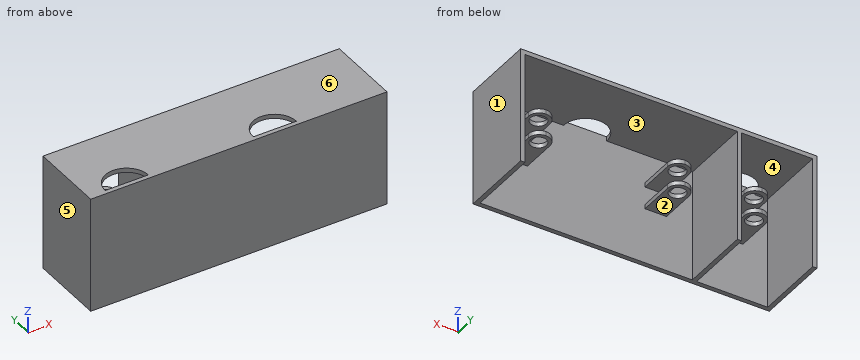
from build123d import *

# Parameters (mm, degrees)
BOSS_EXTRU_1_DEPTH      = 53.6
BOSS_EXTRU_1_DEPTH_BACK = 0.0001
ESQUISSE1_W             = 102.6
ESQUISSE1_H             = 35
ESQUISSE4_W             = 98.6
ESQUISSE4_H             = 51.6
ENL_V_MAT_EXTRU_2_DEPTH = 33
ESQUISSE9_W             = 10
ESQUISSE9_H             = 2
BOSS_EXTRU_3_DEPTH      = 21.5
CONG_2_R                = 5
ESQUISSE10_R            = 3.75
ENL_V_MAT_EXTRU_4_DEPTH = 15
ESQUISSE16_W            = 53.6001
ESQUISSE16_H            = 35
BOSS_EXTRU_5_DEPTH      = 35
ENL_V_MAT_EXTRU_5_DEPTH = 2.1
ESQUISSE19_W            = 33
ESQUISSE19_H            = 51.6001
ENL_V_MAT_EXTRU_6_DEPTH = 33
ENL_V_MAT_EXTRU_7_DEPTH = 2.5
ESQUISSE21_W            = 10
ESQUISSE21_H            = 2
BOSS_EXTRU_6_DEPTH      = 21.75
CONG_3_R                = 5
ESQUISSE22_R            = 3.75
ENL_V_MAT_EXTRU_8_DEPTH = 15


with BuildPart() as part:
    # Esquisse1 → Boss.-Extru.1 (new, two sides: drawn at the far end of the back side and taken through both)
    with BuildSketch(Plane.XY.offset(-BOSS_EXTRU_1_DEPTH_BACK)):
        with Locations((33.832170394, 1.686746988)):
            Rectangle(ESQUISSE1_W, ESQUISSE1_H)
    extrude(amount=BOSS_EXTRU_1_DEPTH + BOSS_EXTRU_1_DEPTH_BACK)

    # Esquisse4 → Enlèv. mat.-Extru.2 (cut)
    with BuildSketch(Plane(origin=(0, 19.186746988, 0), x_dir=(1, 0, 0), z_dir=(0, 1, 0))):
        with Locations((33.832170394, -25.7999)):
            Rectangle(ESQUISSE4_W, ESQUISSE4_H)
    extrude(amount=-ENL_V_MAT_EXTRU_2_DEPTH, mode=Mode.SUBTRACT)

    # Esquisse9 → Boss.-Extru.3 (add)
    with BuildSketch(Plane(origin=(0, -13.813253012, 0), x_dir=(1, 0, 0), z_dir=(0, 1, 0))):
        with Locations((1.532170394, -26.8499)):
            Rectangle(ESQUISSE9_W, ESQUISSE9_H)
        with Locations((1.532170394, -37.2299)):
            Rectangle(ESQUISSE9_W, ESQUISSE9_H)
        with Locations((66.132170394, -26.8499)):
            Rectangle(ESQUISSE9_W, ESQUISSE9_H)
        with Locations((66.132170394, -37.2299)):
            Rectangle(ESQUISSE9_W, ESQUISSE9_H)
    extrude(amount=BOSS_EXTRU_3_DEPTH)

    # Congé2
    cong_2_edges = [part.edges().sort_by_distance(p)[0] for p in [
        (71.132170394, 7.686746988, 37.2299),
        (61.132170394, 7.686746988, 37.2299),
        (71.132170394, 7.686746988, 26.8499),
        (61.132170394, 7.686746988, 26.8499),
        (-3.467829606, 7.686746988, 37.2299),
        (6.532170394, 7.686746988, 37.2299),
        (-3.467829606, 7.686746988, 26.8499),
        (6.532170394, 7.686746988, 26.8499),
    ]]
    fillet(cong_2_edges, radius=CONG_2_R - 0.0001)  # a hair under: the kernel refuses the full size

    # Esquisse10 → Enlèv. mat.-Extru.4 (cut)
    with BuildSketch(Plane(origin=(0, 0, 25.8499), x_dir=(-1, 0, 0), z_dir=(0, 0, -1))):
        with Locations((-66.132170394, 2.186746988)):
            Circle(ESQUISSE10_R)
        with Locations((-1.532170394, 2.186746988)):
            Circle(ESQUISSE10_R)
    extrude(amount=-ENL_V_MAT_EXTRU_4_DEPTH, mode=Mode.SUBTRACT)

    # Esquisse16 → Boss.-Extru.5 (add)
    with BuildSketch(Plane.ZY.offset(17.467829606)):
        with Locations((26.79995, 1.686746988)):
            Rectangle(ESQUISSE16_W, ESQUISSE16_H)
    extrude(amount=BOSS_EXTRU_5_DEPTH)

    # Esquisse18 → Enlèv. mat.-Extru.5 (cut)
    with BuildSketch(Plane.XY.offset(53.6)):
        with BuildLine():
            Line((24.333519225, -13.813253012), (44.330821563, -13.813253012))
            ThreePointArc((44.330821563, -13.813253012), (34.332170394, -3.643205178), (24.333519225, -13.813253012))
        make_face()
    extrude(amount=-ENL_V_MAT_EXTRU_5_DEPTH, mode=Mode.SUBTRACT)

    # Esquisse19 → Enlèv. mat.-Extru.6 (cut)
    with BuildSketch(Plane(origin=(0, 19.186746988, 0), x_dir=(1, 0, 0), z_dir=(0, 1, 0))):
        with Locations((-33.967829606, -25.79995)):
            Rectangle(ESQUISSE19_W, ESQUISSE19_H)
    extrude(amount=-ENL_V_MAT_EXTRU_6_DEPTH, mode=Mode.SUBTRACT)

    # Esquisse20 → Enlèv. mat.-Extru.7 (cut)
    with BuildSketch(Plane.XY.offset(53.6)):
        with BuildLine():
            Line((-24.467829606, -13.813253012), (-44.467829606, -13.813253012))
            ThreePointArc((-44.467829606, -13.813253012), (-34.467829606, -3.813253012), (-24.467829606, -13.813253012))
        make_face()
    extrude(amount=-ENL_V_MAT_EXTRU_7_DEPTH, mode=Mode.SUBTRACT)

    # Esquisse21 → Boss.-Extru.6 (add)
    with BuildSketch(Plane(origin=(0, -13.813253012, 0), x_dir=(1, 0, 0), z_dir=(0, 1, 0))):
        with Locations((-33.967829606, -26.8499)):
            Rectangle(ESQUISSE21_W, ESQUISSE21_H)
        with Locations((-33.967829606, -37.2299)):
            Rectangle(ESQUISSE21_W, ESQUISSE21_H)
    extrude(amount=BOSS_EXTRU_6_DEPTH)

    # Congé3
    cong_3_edges = [part.edges().sort_by_distance(p)[0] for p in [
        (-28.967829606, 7.936746988, 37.2299),
        (-38.967829606, 7.936746988, 37.2299),
        (-38.967829606, 7.936746988, 26.8499),
        (-28.967829606, 7.936746988, 26.8499),
    ]]
    fillet(cong_3_edges, radius=CONG_3_R - 0.0001)  # a hair under: the kernel refuses the full size

    # Esquisse22 → Enlèv. mat.-Extru.8 (cut)
    with BuildSketch(Plane(origin=(0, 0, 25.8499), x_dir=(-1, 0, 0), z_dir=(0, 0, -1))):
        with Locations((33.967829606, 2.186746988)):
            Circle(ESQUISSE22_R)
    extrude(amount=-ENL_V_MAT_EXTRU_8_DEPTH, mode=Mode.SUBTRACT)


solid = part.part
Could you check a few things on this model? Use its own coordinates, in mm. Face numbers are marked on the shaded views. A direction names the side the tool comes from. Give positions to 0.01 mm unless a question says otherwise; leave off trailing zeros. Loops run counter-clockwise (first coordinate to the right, second up) from the corner with the lowest first, then second, coordinate; pieces in that order, holes last. Notation, with made-up numbers: M 89.5,38 L 99.5,38 A24 ccw 99.5,75 Z; hole C -31.75,3 d1. An arc over 180 degrees is marked long. Answer as a JSON object with one key per item and string values.
Q1. Suppose I cut it at B-B, the plane z = 49. List the corners of the cut face in (x, y) for me, plus the area to 3 significant figures.
Values found:
{"outline": "M -52.47,-15.81 L 85.13,-15.81 L 85.13,19.19 L 83.13,19.19 L 83.13,-13.81 L -15.47,-13.81 L -15.47,19.19 L -17.47,19.19 L -17.47,-13.81 L -50.47,-13.81 L -50.47,19.19 L -52.47,19.19 Z", "area": "473 mm²"}
Q2. For P1, Ø3, axis at x = 68.5, y = -7, coming from the -Z side; P2, Ø1, axis at x = 51, y = -9, coming from the -Z side; P3, Ø5, axis at x = 48, z = 9.5, coming from the +Y side, each with a flat end and sliding along its axis, tell me the tip position at first contact or that it passes through.
Values found:
{"P1": "stops at z = 25.85", "P2": "stops at z = 51.6", "P3": "stops at y = -13.81"}
Q3. If I drill on probe 1 along X at (y, z) = (12, 46.5); probe 2 along Z at (x, y) = (6, 1.5); probe 3 along Z at (x, y) = (55.5, -3), over which ranges is the centre line in solid material (lowest first)? Write a range as [from, to].
Values found:
{"probe 1": "x = [-52.47, -50.47], [-17.47, -15.47], [83.13, 85.13]", "probe 2": "z = [25.85, 27.85], [36.23, 38.23], [51.6, 53.6]", "probe 3": "z = [51.6, 53.6]"}
Q4. For the marked faces 1 and 2, which set-ups out of +Z, -Z, +X, -X, +Y, -Y let a thin tool reach every point of the face, with its end or its side?
Values found:
{"face 1": "+Z, -Z, +X, +Y, -Y", "face 2": "-Z, +Y"}
Q5. Suppose I cut it at D-D, the plane x = 3.5. List the corners of the cut face in (y, z) for me, plus the area to 3 significant figures.
Values found:
{"outline": "M -15.81,0 L -13.81,0 L -13.81,25.85 L -1.01,25.85 L -1.01,27.85 L -13.81,27.85 L -13.81,36.23 L -1.01,36.23 L -1.01,38.23 L -13.81,38.23 L -13.81,51.6 L 19.19,51.6 L 19.19,53.6 L -15.81,53.6 Z; M 5.38,25.85 L 7.28,25.85 L 7.28,27.85 L 5.38,27.85 Z; M 5.38,36.23 L 7.28,36.23 L 7.28,38.23 L 5.38,38.23 Z", "area": "232 mm²"}
Q6. If we mould it in two halves opening along X, with no side actions, what happens to the marked faces 3, 4, 5 and 6? For each: pulls with the +X half, pulls with the -X half, needs draft (parallel to the pull), parting line crosses it, or undercut.
Values found:
{"face 3": "undercut", "face 4": "undercut", "face 5": "pulls with the -X half", "face 6": "needs draft"}
Q7. Suppose I cut it at C-C, the plane x = 64.5. List the corners of the cut face in (y, z) for me.
Values found:
{"outline": "M -15.81,0 L -13.81,0 L -13.81,25.85 L -1.19,25.85 L -1.19,27.85 L -13.81,27.85 L -13.81,36.23 L -1.19,36.23 L -1.19,38.23 L -13.81,38.23 L -13.81,51.6 L 19.19,51.6 L 19.19,53.6 L -15.81,53.6 Z; M 5.56,25.85 L 7.41,25.85 L 7.41,27.85 L 5.56,27.85 Z; M 5.56,36.23 L 7.41,36.23 L 7.41,38.23 L 5.56,38.23 Z"}
Q8. Suppose I cut it at A-A, the plane x = 30.5. List the corners of the cut face in (y, z) for me, plus the area to 3 significant figures.
Values found:
{"outline": "M -15.81,0 L -13.81,0 L -13.81,53.6 L -15.81,53.6 Z; M -4.41,51.6 L 19.19,51.6 L 19.19,53.6 L -4.41,53.6 Z", "area": "154 mm²"}
